```python
from build123d import *

# Parameters (mm, degrees)
SKETCH1_W               = 80
SKETCH1_H               = 54.5
SKETCH1_R               = 19.25
BOSS_EXTRUDE1_DEPTH     = 1.27
SHELL4_T                = 5
SKETCH7_W               = 90
SKETCH7_H               = 5
BOSS_EXTRUDE4_DEPTH     = 20
SKETCH1_5_R             = 19.25
CUT_EXTRUDE3_DEPTH      = 61.745884634
CUT_EXTRUDE3_DEPTH_BACK = 61.745884634


with BuildPart() as part:
    # Sketch1 → Boss-Extrude1 (new body)
    with BuildSketch(Plane(origin=(0, 0, 0), x_dir=(1, 0, 0), z_dir=(0, 1, 0))):
        Rectangle(SKETCH1_W, SKETCH1_H)
        Circle(SKETCH1_R, mode=Mode.SUBTRACT)
        Circle(SKETCH1_R)
    extrude(amount=-BOSS_EXTRUDE1_DEPTH)

    # Shell4
    shell4_openings = [part.faces().sort_by_distance(p)[0] for p in [
        (0, -1.27, 0),
    ]]
    offset(amount=SHELL4_T, openings=shell4_openings, kind=Kind.INTERSECTION)

    # Sketch7 → Boss-Extrude4 (add)
    with BuildSketch(Plane(origin=(0, 5, 0), x_dir=(1, 0, 0), z_dir=(0, 1, 0))):
        with Locations((0, 29.75)):
            Rectangle(SKETCH7_W, SKETCH7_H)
        with Locations((0, -29.75)):
            Rectangle(SKETCH7_W, SKETCH7_H)
    extrude(amount=BOSS_EXTRUDE4_DEPTH)

    # Sketch1_5 → Cut-Extrude3 (cut, two sides)
    with BuildSketch(Plane(origin=(0, 0, 0), x_dir=(1, 0, 0), z_dir=(0, 1, 0))) as cut_extrude3_sk:
        with Locations(Location((0, 0, 0), (0, 0, 270))):
            Circle(SKETCH1_5_R)
    cut_extrude3 = extrude(amount=CUT_EXTRUDE3_DEPTH, mode=Mode.SUBTRACT)
    cut_extrude3 = cut_extrude3 + extrude(cut_extrude3_sk.sketch, amount=-CUT_EXTRUDE3_DEPTH_BACK, mode=Mode.SUBTRACT)

    # Mirror1: Cut-Extrude3 across plane
    add(cut_extrude3.mirror(Plane.XY), mode=Mode.SUBTRACT)


solid = part.part
```
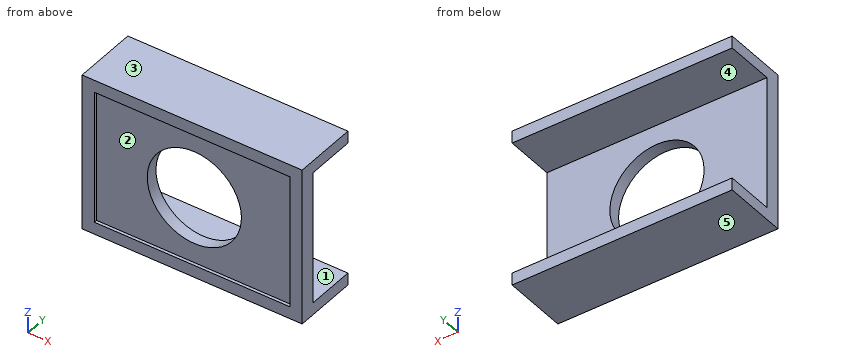
Design review of the part built by this model. Coordinates are the model's own, in mm. Face numbers are marked on the shaded views. A direction names the side the tool comes from. Give positions to 0.01 mm unless a question says otherwise; leave off trailing zeros. Loops run counter-clockwise (first coordinate to the right, second up) from the corner with the lowest first, then second, coordinate; pieces in that order, holes last. Notation, with made-up numbers: M 30,-11 L 71,-11 A31 ccw 71,27 Z; hole C -4,43.25 d1. An arc over 180 degrees is marked long. Return JSON: item names as keys, results as strings. Group by question number.
Item 1: We need section B-B (x = 0). Give the boundary of the cut face in (y, z), and give its area (3 significant figures).
Item 2: We need section C-C (z = 0). Give the boundary of the cut face in (x, y), and give its area (3 significant figures).
Item 3: Insertion check: pin 1 Ø16.5 at (x, z) = (5.5, -10) entering from +Y; pin 2 Ø10 at (x, z) = (14, -0.5) entering from -Y (3 decimals); pin 3 Ø6 at (x, z) = (-23.5, -18.5) entering from -Y. Each pin has a flat end and moves straight along its axis. Give the tip position at first contact, or say it passes through.
Item 4: Mouldability with a two-part tool opening along Z and no side actions: class the marked faces 3, 4 and 5 as released by +Z, released by -Z, zero draft, split by the parting line, or undercut.
Item 5: We need section A-A (y = 15.75). Give the boundary of the cut face in (x, z), and give its area (3 significant figures).
Item 6: For probe 1 along Z at (x, y) = (0, 2.5); probe 2 along X at (y, z) = (1.8, 0); probe 3 along Z at (x, y) = (5.5, 17.75), list the stretches that pass through material, from the lowest coordinate up.
Item 7: We need section D-D (y = 1). Give the boundary of the cut face in (x, z), and give its area (3 significant figures).
Item 8: Tool access review of the marked faces 1 and 2: name each direction out of +Z, -Z, +X, -X, +Y, -Y from which nothing blocks a thin tool from reaching the whole face with its end or side.
Output:
{
 "1": {"outline": "M -1.27,-32.25 L 25,-32.25 L 25,-27.25 L 5,-27.25 L 5,-19.25 L 0,-19.25 L 0,-27.25 L -1.27,-27.25 Z; M -1.27,27.25 L 0,27.25 L 0,19.25 L 5,19.25 L 5,27.25 L 25,27.25 L 25,32.25 L -1.27,32.25 Z", "area": "343 mm^2"},
 "2": {"outline": "M -45,-1.27 L -40,-1.27 L -40,0 L -19.25,0 L -19.25,5 L -45,5 Z; M 19.25,0 L 40,0 L 40,-1.27 L 45,-1.27 L 45,5 L 19.25,5 Z", "area": "270 mm^2"},
 "3": {"pin 1": "stops at y = 5", "pin 2": "passes through", "pin 3": "stops at y = 0"},
 "4": {"face 3": "released by +Z", "face 4": "undercut", "face 5": "released by -Z"},
 "5": {"outline": "M -45,-32.25 L 45,-32.25 L 45,-27.25 L -45,-27.25 Z; M -45,27.25 L 45,27.25 L 45,32.25 L -45,32.25 Z", "area": "900 mm^2"},
 "6": {"probe 1": "z = -32.25 to -19.25, 19.25 to 32.25", "probe 2": "x = -45 to -19.25, 19.25 to 45", "probe 3": "z = -32.25 to -27.25, 27.25 to 32.25"},
 "7": {"outline": "M -45,-32.25 L 45,-32.25 L 45,32.25 L -45,32.25 Z; hole C 0,0 d38.5", "area": "4,640 mm^2"},
 "8": {"face 1": "+X, -X, +Y", "face 2": "-Y"}
}
